Part model, mm, in its own coordinate system. A direction names the side the tool comes from. Coordinates: 2 decimals unless noted, no trailing zeros. Order: outer loops, then holes, each group sorted by start corner. A loop starts at its lowest first (then second) coordinate and runs counter-clockwise, first axis right, second up. Notation, with made-up numbers: (-9.75, 36) - (40.25, 36) arc R26 cw to (40.25, 60) - close; hole circle Ø8 at (47.5, 50). An arc over 180 degrees is marked (long way). Use a Markdown table: item, result. Add a question column.
1) Wall check: L1, parallel to Z at x = 7.5, y = 0.3; L2, parallel to X at y = 7.5, z = 108.5. Give the ranges that are in metal, low to high. Write a range as [from, to].
2) Saw through at B-B on x = 7.5. List the corners of the cut face in (y, z), then the cut area to 3 significant figures.
3) Saw through at D-D on z = 80.5. List the corners of the cut face in (x, y).
4) Saw through at C-C on y = 7.5. List the corners of the cut face in (x, z), then the cut area to 3 significant figures.
5) Tool access for faces 1 (the face through (8, 1.5, 69)), 2 (the face through (7.79, 0.74, 117.82)): list every direction of +Z, -Z, +X, -X, +Y, -Y with a clear straight run to the whole face (end or side of a thin tool).
6) Drop flat-ended pins along their axis: P1, Ø1, axis at x = 5.5, z = 122.5, coming from the +Y side; P2, Ø4, axis at y = 5.5, z = 56, coming from the +X side. Give the stop position or say it passes through.
7) Saw through at A-A on z = 130. List the corners of the cut face in (x, y), then the cut area to 4 significant figures.
8) Two-plate mould, pull along Z, no slides. Class faces 3 (the face through (0.74, 8.919, 8.452)), 4 (the face through (4, 1, 0)), 5 (the face through (0, 7, 69)): +Z half, -Z half, draft (parallel to the pull), parting line (faces both ways), or undercut.
```python
from build123d import *

# Parameters (mm, degrees)
EXTRUDE_1_DEPTH     = 140
SKETCH_2_R          = 2.1
CUT_EXTRUDE_1_DEPTH = 140
SKETCH_3_R          = 2.2
CUT_EXTRUDE_2_DEPTH = 140


with BuildPart() as part:
    # ｽｹｯﾁ1 → ﾎﾞｽ - 押し出し1 (new body)
    with BuildSketch(Plane.XY):
        Polygon((0, 0), (0, 15), (1.5, 15), (1.5, 1.5), (15, 1.5), (15, 0), align=None)
    extrude(amount=EXTRUDE_1_DEPTH)

    # ｽｹｯﾁ2 → ｶｯﾄ - 押し出し1 (cut)
    with BuildSketch(Plane.ZY):
        with Locations((130, 7.5)):
            Circle(SKETCH_2_R)
        with Locations((10, 7.5)):
            Circle(SKETCH_2_R)
    extrude(amount=-CUT_EXTRUDE_1_DEPTH, mode=Mode.SUBTRACT)

    # ｽｹｯﾁ3 → ｶｯﾄ - 押し出し2 (cut)
    with BuildSketch(Plane(origin=(0, 0, 0), x_dir=(-1, 0, 0), z_dir=(0, -1, 0))):
        with Locations((-7.5, -120)):
            Circle(SKETCH_3_R)
        with Locations((-7.5, -20)):
            Circle(SKETCH_3_R)
    extrude(amount=-CUT_EXTRUDE_2_DEPTH, mode=Mode.SUBTRACT)


solid = part.part
```
Results are:
| question | item | result |
|---|---|---|
| 1 | L1 | [0, 17.8], [22.2, 117.8], [122.2, 140] |
| 1 | L2 | [0, 1.5] |
| 2 | outline | (0, 0) - (1.5, 0) - (1.5, 17.8) - (0, 17.8) - close; (0, 22.2) - (1.5, 22.2) - (1.5, 117.8) - (0, 117.8) - close; (0, 122.2) - (1.5, 122.2) - (1.5, 140) - (0, 140) - close |
| 2 | area | 197 mm2 |
| 3 | outline | (0, 0) - (15, 0) - (15, 1.5) - (1.5, 1.5) - (1.5, 15) - (0, 15) - close |
| 4 | outline | (0, 0) - (1.5, 0) - (1.5, 7.9) - (0, 7.9) - close; (0, 12.1) - (1.5, 12.1) - (1.5, 127.9) - (0, 127.9) - close; (0, 132.1) - (1.5, 132.1) - (1.5, 140) - (0, 140) - close |
| 4 | area | 197 mm2 |
| 5 | face 1 | +Z, -Z, +X, +Y |
| 5 | face 2 | +Y, -Y |
| 6 | P1 | y = 1.5 |
| 6 | P2 | x = 1.5 |
| 7 | outline | (0, 0) - (15, 0) - (15, 1.5) - (1.5, 1.5) - (1.5, 5.4) - (0, 5.4) - close; (0, 9.6) - (1.5, 9.6) - (1.5, 15) - (0, 15) - close |
| 7 | area | 36.45 mm2 |
| 8 | face 3 | undercut |
| 8 | face 4 | -Z half |
| 8 | face 5 | draft |
